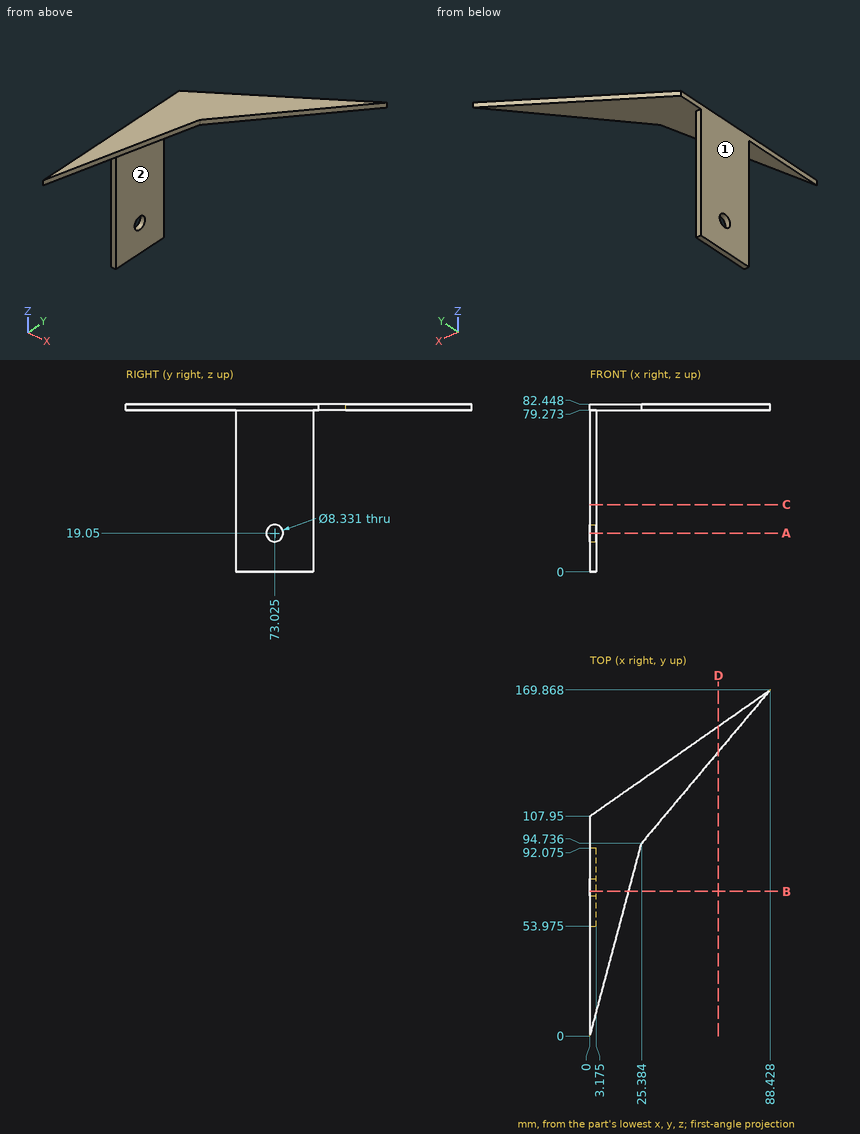
Check sheet for the drawn part. Datum: minimum x, y, z corner. Units: mm. A direction names the side the tool comes from. Round coordinates to 2 decimals unless told otherwise and drop trailing zeros. Write each loop counter-clockwise with the first axis right and the second up, starting at its lowest first coordinate (ties: lowest second). Pieces come first, ordered by that corner, then holes. Notation, with made-up numbers: (38.25, -4.5) -> (65.25, -4.5) arc R29 cw to (65.25, 26.5) -> close; hole circle Ø8 at (52, -26.5). An arc over 180 degrees is marked (long way). Write each question's results on one line, items separated by ' | '.
Q1. Sectioned sample at B-B, the plane y = 71. Record the boundary of the cut face in (x, z) (1 decimal), and give its area (3 significant figures).
Derived:
outline: (0, 0) -> (3.2, 0) -> (3.2, 15.4) -> (0, 15.4) -> close; (0, 22.7) -> (3.2, 22.7) -> (3.2, 79.3) -> (19, 79.3) -> (19, 82.4) -> (0, 82.4) -> close | area: 289 mm²
Q2. Sectioned sample at A-A, the plane z = 19.05. Record the boundary of the cut face in (x, y) (1 decimal).
Derived:
outline: (0, 54) -> (3.2, 54) -> (3.2, 68.9) -> (0, 68.9) -> close; (0, 77.2) -> (3.2, 77.2) -> (3.2, 92.1) -> (0, 92.1) -> close
Q3. Thickness scan on probe 1 along Y at (x, z) = (0.95, 19.05) (1 decimal); probe 2 along X at (y, z) = (79, 22.5) (1 decimal); probe 3 along Z at (x, y) = (44.5, 129.5). Record the ranges inside material, lowest first.
Derived:
probe 1: y = 54 to 68.9, 77.2 to 92.1 | probe 2: x = 0 to 3.2 | probe 3: z = 79.27 to 82.45
Q4. Sectioned sample at C-C, the plane z = 33. Record the boundary of the cut face in (x, y) (1 decimal), and give its area (3 significant figures).
Derived:
outline: (0, 54) -> (3.2, 54) -> (3.2, 92.1) -> (0, 92.1) -> close | area: 121 mm²
Q5. Go/stop test with flat-tipped pins: pin 1 Ø1 at (x, z) = (1, 57.5) entering from +Y (1 decimal); pin 2 Ø3 at (y, z) = (55.5, 68) entering from -X; pin 3 Ø2.5 at (x, z) = (1.5, 20) entering from -Y (1 decimal); pin 4 Ø7.5 at (y, z) = (73.025, 19.05) entering from +X. Record where each tip stops, or that it passes through.
Derived:
pin 1: stops at y = 92.1 | pin 2: stops at x = 0 | pin 3: stops at y = 54 | pin 4: passes through
Q6. Access from +Z, -Z, +X, -X, +Y, -Y to the whole of each face (thin tool, end or side, straight path). Record for the marked faces 1 and 2.
Derived:
face 1: +Z, -Z, -X, +Y, -Y | face 2: -Z, +X, +Y, -Y
Q7. Sectioned sample at D-D, the plane x = 63. Record the boundary of the cut face in (y, z) (1 decimal).
Derived:
outline: (139.6, 79.3) -> (152.1, 79.3) -> (152.1, 82.4) -> (139.6, 82.4) -> close
